CAD build for the part. Positions are in the model's coordinates, mm. A direction names the side the tool comes from. Coordinates: 2 decimals unless noted, no trailing zeros. Loops run counter-clockwise (first coordinate to the right, second up) from the corner with the lowest first, then second, coordinate; pieces in that order, holes last. Notation, with made-up numbers: (-25, -22.5) -> (-20, -22.5) arc R25 ccw to (-20, 11.5) -> close; hole circle Ø2 at (-15, 1.25). An arc over 180 degrees is marked (long way). Return JSON: item names as keys, results as strings. Group by question number.
(1) Mould opens along X. For faces 3 (the face through (0, -6, 20)), 4 (the face through (13, 0, 35)), 5 (the face through (10.502, -3.219, 53.438)) say: pulls with the +X half, pulls with the -X half, needs draft (parallel to the pull), parting line crosses it, or undercut.
(2) Saw through at C-C on x = 3.5. Write the cut outline in (y, z).
(3) Saw through at A-A on x = 12.7. Give the number of separate pieces and of enclosed holes in the cut face, then the cut area to 3 significant figures.
(4) Saw through at D-D on z = 19. Write the cut outline in (x, y).
(5) Flat gauge pins, fed straight in: pin 1 Ø3 at (x, z) = (6, 37) entering from -Y; pin 2 Ø5 at (x, y) = (23, -29.5) entering from +Z. Where does each tip first touch, or does it go through?
(6) Saw through at B-B on y = -27. Write the cut outline in (x, z), then the cut area to 3 significant figures.
(7) Tool access for faces 1 (the face through (13, -6.35, 38)), 2 (the face through (13, -18, 0)): list every direction of +Z, -Z, +X, -X, +Y, -Y with a clear straight run to the whole face (end or side of a thin tool).
(8) Probe L1, parallel to Z at x = 13.25, y = -19; L2, parallel to Y at x = 4.25, z = 30; L3, parallel to Y at x = 12.7, z = 2. List the from-to ranges inside material, lowest first.
```python
from build123d import *

# Parameters (mm, degrees)
F0_W     = 12.7
F0_H     = 6.35
F1_DEPTH = 38.1
F0_H_2   = 57.15
F2_DEPTH = 6.35
F3_R     = 5.08
F5_D     = 9.525
F6_D     = 9.525


# Not quite as in the source:
# - a length typed as a fraction of an inch, garbled in the dataset ("3 / 203.2 mm" for 3/8 in), is restored


with BuildPart() as f1:
    # F0 (on Front) → F1 (new body)
    with BuildSketch(Plane.XZ):
        with Locations((6.35, 3.175)):
            Rectangle(F0_W, F0_H)
        with Locations((19.05, 3.175)):
            Rectangle(F0_W, F0_H)
    extrude(amount=F1_DEPTH)

    # F0 (on Front) → F2 (join)
    with BuildSketch(Plane.XZ):
        with Locations((6.35, 3.175)):
            Rectangle(F0_W, F0_H)
        with Locations((19.05, 3.175)):
            Rectangle(F0_W, F0_H)
        with Locations((6.35, 34.925)):
            Rectangle(F0_W, F0_H_2)
        with Locations((19.05, 34.925)):
            Rectangle(F0_W, F0_H_2)
    extrude(amount=F2_DEPTH)

    # F3
    f3_edges = [f1.edges().sort_by_distance(p)[0] for p in [
        (12.7, -6.35, 6.35),
        (12.7, 0, 0),
    ]]
    fillet(f3_edges, radius=F3_R)

    # F5 (through all)
    with Locations(Plane.XY.offset(6.35)):
        with Locations((12.7, -24.765)):
            Hole(F5_D / 2)

    # F6 (through all)
    with Locations(Plane(origin=(0, 0, 0), x_dir=(1, 0, 0), z_dir=(0, 1, 0))):
        with Locations((12.7, -49.2125)):
            Hole(F6_D / 2)


solid = f1.part
```
Geometry results:
{
 "1": {"face 3": "pulls with the -X half", "face 4": "needs draft", "face 5": "undercut"},
 "2": {"outline": "(-38.1, 0) -> (-5.08, 0) arc R5.08 ccw to (0, 5.08) -> (0, 63.5) -> (-6.35, 63.5) -> (-6.35, 11.43) arc R5.08 cw to (-11.43, 6.35) -> (-38.1, 6.35) -> close"},
 "3": {"separate pieces": "3", "enclosed holes": "0", "area": "484 mm²"},
 "4": {"outline": "(0, -6.35) -> (25.4, -6.35) -> (25.4, 0) -> (0, 0) -> close"},
 "5": {"pin 1": "y = -6.35", "pin 2": "z = 6.35"},
 "6": {"outline": "(0, 0) -> (8.49, 0) -> (8.49, 6.35) -> (0, 6.35) -> close; (16.91, 0) -> (25.4, 0) -> (25.4, 6.35) -> (16.91, 6.35) -> close", "area": "108 mm²"},
 "7": {"face 1": "+Z, +X, -X, -Y", "face 2": "-Z, +X, -X, +Y, -Y"},
 "8": {"L1": "0 to 6.35", "L2": "-6.35 to 0", "L3": "-38.1 to -29.53, -20 to -1.04"}
}
